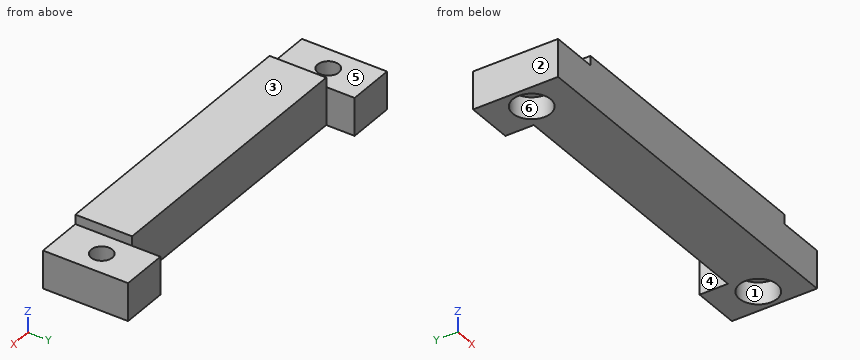
Autodesk Inventor part; units mm, degrees
ref_plane "YZ Plane" through (0, 0, 0) normal (1, 0, 0) x (0, 1, 0)
ref_plane "XZ Plane" through (0, 0, 0) normal (0, 1, 0) x (-1, 0, 0)
ref_plane "XY Plane" through (0, 0, 0) normal (0, 0, 1) x (1, 0, 0)
sketch "Skizze1" plane through (0, 0, 0) normal (0, 0, 1) x (1, 0, 0)
  line L0 (-40, 9) -> (40, 9)
  line L1 (40, 9) -> (40, -9)
  line L2 (40, -9) -> (-40, -9)
  line L3 (-40, -9) -> (-40, 9)
  line L4 (-40, 9) -> (40, -9) construction
  line L5 (40, 9) -> (-40, -9) construction
  point P0 (0, 0)
  dimension "Breite" = 80
  dimension "d1" = 18
extrude "Extrusion1" add sketch "Skizze1" along normal blind 10
sketch "Skizze2" plane through (0, 0, 10) normal (0, 0, 1) x (1, 0, 0)
  line L0 (-56, 0) -> (56, 0)
  line L1 (0, -12.6) -> (0, 12.6)
  line L2 (40, 9) -> (-40, 9)
  line L3 (-40, 9) -> (-40, -9)
  line L4 (-40, -9) -> (40, -9)
  line L5 (40, -9) -> (40, 9)
  line L6 (30, 3) -> (-30, 3)
  line L7 (-30, 3) -> (-30, 9)
  line L8 (-30, 9) -> (30, 9)
  line L9 (30, 9) -> (30, 3)
  line L10 (30, 3) -> (-30, 9) construction
  line L11 (-30, 3) -> (30, 9) construction
  point P0 (0, 0)
  point P1 (0, 6)
  dimension "d4" = 60
  dimension "d5" = 6
extrude "Extrusion2" cut sketch "Skizze2" against normal through all contours L6 L7 L2 L1 | L1 L2 L9 L6
sketch "Skizze3" plane through (0, 0, 10) normal (0, 0, 1) x (1, 0, 0)
  line L0 (-30, 9) -> (-40, 9)
  line L1 (-30, 9) -> (-40, 9)
  line L2 (-40, 9) -> (-40, -9)
  line L3 (-40, -9) -> (-30, -9)
  line L4 (-30, -9) -> (-30, 9)
  point P0 (0, 0)
extrude "Extrusion3" cut sketch "Skizze3" against normal blind 2
sketch "Skizze4" plane through (0, 0, 10) normal (0, 0, 1) x (1, 0, 0)
  line L0 (40, 9) -> (30, 9)
  line L1 (30, 9) -> (30, -9)
  line L2 (30, -9) -> (40, -9)
  line L3 (40, -9) -> (40, 9)
  point P0 (0, 0)
extrude "Extrusion4" cut sketch "Skizze4" against normal blind 2
sketch "Skizze5" plane through (0, 0, 0) normal (0, 0, -1) x (-1, 0, 0)
  line L0 (0, -12.6) -> (0, 12.6)
  line L1 (-30, 9) -> (-40, 9)
  point P0 (0, 0)
  point P1 (-35, 0)
  point P2 (35, 0)
  dimension "d12" = 9
hole "Bohrung1" at (35, 0, 0) at (-35, 0, 0) direction (0, 0, 1) diameter 4.5 end through all counterbore diameter 8 counterbore depth 4.6
properties part number "ABI_KastenSchnitt"
Check sheet for the modelled part. Datum: model origin and axes. Units: mm. Face numbers are marked on the shaded views. A direction names the side the tool comes from. Give positions to 0.01 mm unless a question says otherwise; leave off trailing zeros. Write each loop counter-clockwise with the first axis right and the second up, starting at its lowest first coordinate (ties: lowest second). Pieces come first, ordered by that corner, then holes. Notation, with made-up numbers: (-4.75, 24.5) -> (46.25, 24.5) arc R29 ccw to (46.25, 54.5) -> close; hole circle Ø5 at (24.5, 2.5). An arc over 180 degrees is marked (long way). Use one line per item in the form item = value. Start each with the question number.
1. Mould release check, pull along X, two halves, no side actions. Record for the marked faces 1, 2 and 3: pulls with the +X half, pulls with the -X half, needs draft (parallel to the pull), parting line crosses it, or undercut.
2. Access from +Z, -Z, +X, -X, +Y, -Y to the whole of each face (thin tool, end or side, straight path). Record for the marked faces 4, 5 and 6.
3. Thickness scan on line 1 along X through (y, z) = (0, 6.45); line 2 along Y through (x, z) = (35, 3.55); line 3 along X through (y, z) = (-2.5, 3). Record the ranges inside material, lowest first. Write a range as from..to.
4. Section check C-C (z = 6). Record the cut outline in (x, y).
5. Section check B-B (y = 0). Record the cut outline in (x, z).
6. Section check D-D (y = 6.75). Record the cut outline in (x, z), and give its area (3 significant figures).
7. Go/stop test with flat-tipped pins: P1, Ø6, axis at x = -35, y = 0, coming from the -Z side; P2, Ø9, axis at x = 35, y = 0, coming from the +Z side; P3, Ø1.6, axis at y = -4, z = 9.5, coming from the +X side. Record where each tip stops, or that it passes through.
8. Section check A-A (x = 35). Record the cut outline in (y, z).
Conclusion:
q1.face_1 = undercut
q1.face_2 = pulls with the -X half
q1.face_3 = needs draft
q2.face_4 = +Z, -Z, +Y
q2.face_5 = +Z, -X, +Y, -Y
q2.face_6 = -Z
q3.line_1 = -40..-37.25, -32.75..32.75, 37.25..40
q3.line_2 = -9..-4, 4..9
q3.line_3 = -40..-38.12, -31.88..31.88, 38.12..40
q4.outline = (-40, -9) -> (40, -9) -> (40, 9) -> (30, 9) -> (30, 3) -> (-30, 3) -> (-30, 9) -> (-40, 9) -> close; hole circle Ø4.5 at (-35, 0); hole circle Ø4.5 at (35, 0)
q5.outline = (-40, 0) -> (-39, 0) -> (-39, 4.6) -> (-37.25, 4.6) -> (-37.25, 8) -> (-40, 8) -> close; (-32.75, 4.6) -> (-31, 4.6) -> (-31, 0) -> (31, 0) -> (31, 4.6) -> (32.75, 4.6) -> (32.75, 8) -> (30, 8) -> (30, 10) -> (-30, 10) -> (-30, 8) -> (-32.75, 8) -> close; (37.25, 4.6) -> (39, 4.6) -> (39, 0) -> (40, 0) -> (40, 8) -> (37.25, 8) -> close
q6.outline = (-40, 0) -> (-30, 0) -> (-30, 8) -> (-40, 8) -> close; (30, 0) -> (40, 0) -> (40, 8) -> (30, 8) -> close
q6.area = 160 mm²
q7.P1 = 4.6
q7.P2 = 8
q7.P3 = 30
q8.outline = (-9, 0) -> (-4, 0) -> (-4, 4.6) -> (-2.25, 4.6) -> (-2.25, 8) -> (-9, 8) -> close; (2.25, 4.6) -> (4, 4.6) -> (4, 0) -> (9, 0) -> (9, 8) -> (2.25, 8) -> close
